Could you check a few things on this drawing? It's one solid part, dimensions in mm from its lowest x, y, z. A direction names the side the tool comes from. Give positions to 0.01 mm unless a question says otherwise; leave off trailing zeros. Loops run counter-clockwise (first coordinate to the right, second up) from the corner with the lowest first, then second, coordinate; pieces in that order, holes last.
Q1. Suppose I cut it at A-A (z = 400). List the corners of the cut face in (x, y) for me, and give its area (3 significant figures).
Q2. Suppose I cut it at D-D (z = 107). List the corners of the cut face in (x, y) for me.
Q3. Suppose I cut it at B-B (x = 923). List the corners of the cut face in (y, z) for me, and give its area (3 significant figures).
Q4. For the marked faces 4 and 5, which set-ups out of +Z, -Z, +X, -X, +Y, -Y let a thin tool reach every point of the face, with its end or its side?
Q5. Suppose I cut it at C-C (y = 19.5). List the corners of the cut face in (x, z) for me, and give its area (3 significant figures).
Q6. Thinking about a two-plate mould opening in Z: for the marked faces 1, 2 and 3, which applies, pulls with the +Z half, pulls with the -Z half, needs draft (parallel to the pull), parting line crosses it, or undercut?
Q7. I need wall thicknesses on probe 1 along Z at (x, y) = (67.5, 60); probe 2 along X at (y, z) = (62, 65); probe 3 along Y at (x, z) = (609, 449). Which ranges of each line are inside material? Lowest first, please.
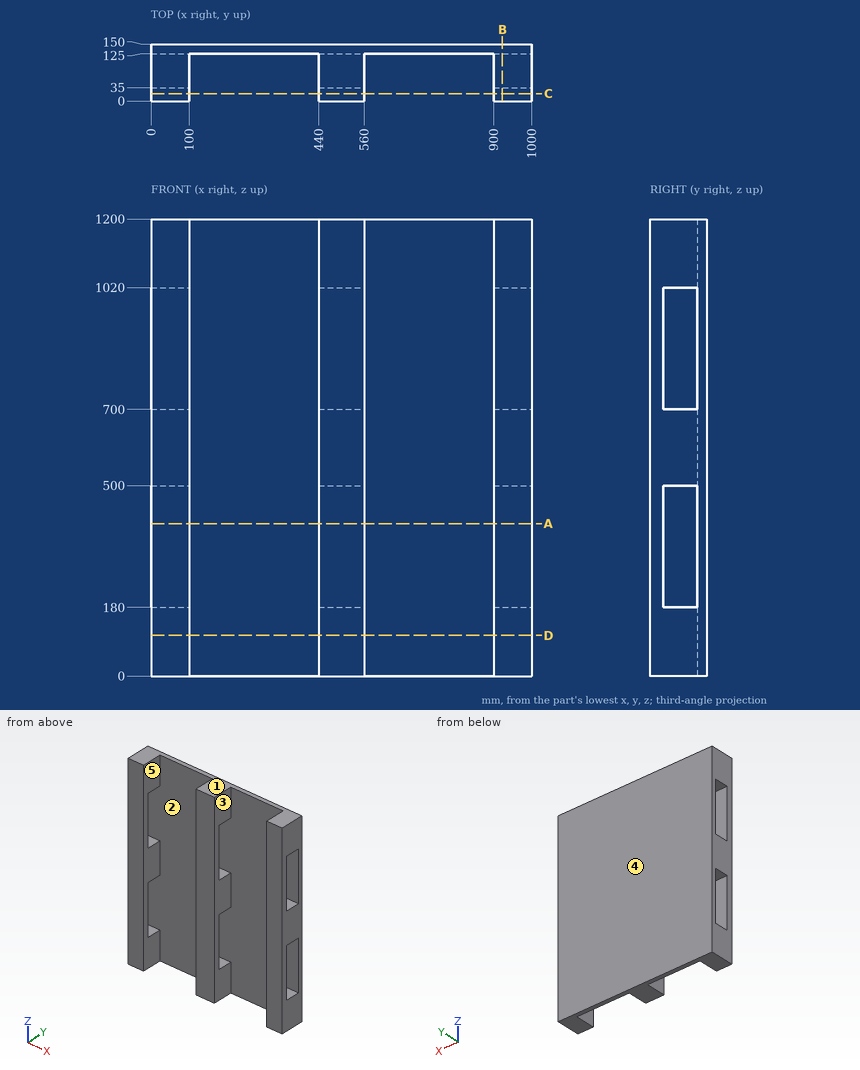
Solutions:
1. outline: (0, 0) - (100, 0) - (100, 35) - (0, 35) - close; (0, 125) - (1000, 125) - (1000, 150) - (0, 150) - close; (440, 0) - (560, 0) - (560, 35) - (440, 35) - close; (900, 0) - (1000, 0) - (1000, 35) - (900, 35) - close
1. area: 36,200 mm2
2. outline: (0, 0) - (100, 0) - (100, 125) - (440, 125) - (440, 0) - (560, 0) - (560, 125) - (900, 125) - (900, 0) - (1000, 0) - (1000, 150) - (0, 150) - close
3. outline: (0, 0) - (150, 0) - (150, 1200) - (0, 1200) - close; hole (35, 180) - (125, 180) - (125, 500) - (35, 500) - close; hole (35, 700) - (125, 700) - (125, 1020) - (35, 1020) - close
3. area: 122,000 mm2
4. face 4: +Z, -Z, +X, -X, +Y
4. face 5: +Z, -Z, -Y
5. outline: (0, 0) - (100, 0) - (100, 1200) - (0, 1200) - close; (440, 0) - (560, 0) - (560, 1200) - (440, 1200) - close; (900, 0) - (1000, 0) - (1000, 1200) - (900, 1200) - close
5. area: 384,000 mm2
6. face 1: pulls with the +Z half
6. face 2: undercut
6. face 3: needs draft
7. probe 1: z = 0 to 180, 500 to 700, 1020 to 1200
7. probe 2: x = 0 to 100, 440 to 560, 900 to 1000
7. probe 3: y = 125 to 150
